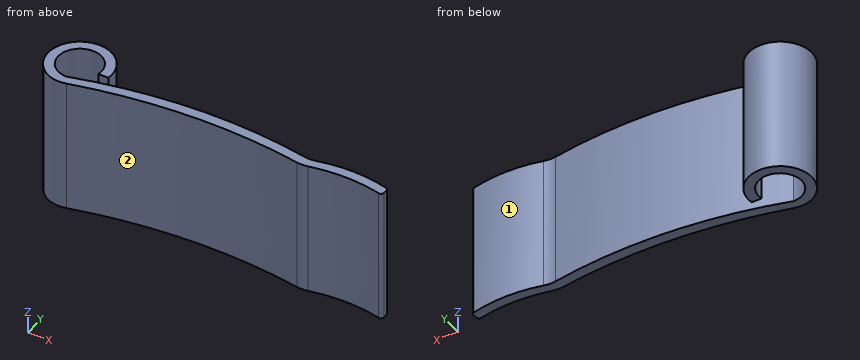
from build123d import *

# Parameters (mm, degrees)
BOSS_EXTRUDE1_DEPTH = 11.811
FILLET1_R           = 2.54
FILLET2_R           = 2.54
FILLET3_R           = 2.54
FILLET4_R           = 0.254


with BuildPart() as part:
    # Sketch1 → Boss-Extrude1 (new body)
    with BuildSketch(Plane.XY):
        with BuildLine():
            Line((28.176033565, -1.032201382), (28.176033565, -1.921201382))
            ThreePointArc((28.176033565, -1.921201382), (24.613856271, -1.460610767), (21.051678976, -1.921201382))
            ThreePointArc((21.051678976, -1.921201382), (10.446405641, -1.176341171), (-0.061202039, -2.794))
            ThreePointArc((-0.061202039, -2.794), (-1.825200311, 2.116323585), (2.772672487, -0.349955666))
            Line((2.772672487, -0.349955666), (1.874071212, -0.34188023))
            ThreePointArc((1.874071212, -0.34188023), (-1.220193255, 1.462926321), (0, -1.905))
            ThreePointArc((0, -1.905), (10.542698007, -0.186192099), (21.191033565, -1.032201382))
            ThreePointArc((21.191033565, -1.032201382), (24.683533565, -0.542543055), (28.176033565, -1.032201382))
        make_face()
    extrude(amount=BOSS_EXTRUDE1_DEPTH)

    # Fillet1
    fillet1_edges = [part.edges().sort_by_distance(p)[0] for p in [
        (-0.061202039, -2.794, 5.9055),
    ]]
    fillet(fillet1_edges, radius=FILLET1_R)

    # Fillet2
    fillet2_edges = [part.edges().sort_by_distance(p)[0] for p in [
        (21.051678976, -1.921201382, 5.9055),
    ]]
    fillet(fillet2_edges, radius=FILLET2_R)

    # Fillet3
    fillet3_edges = [part.edges().sort_by_distance(p)[0] for p in [
        (21.191033565, -1.032201382, 5.9055),
    ]]
    fillet(fillet3_edges, radius=FILLET3_R)

    # Fillet4
    fillet4_edges = [part.edges().sort_by_distance(p)[0] for p in [
        (28.176033565, -1.032201382, 5.9055),
        (28.176033565, -1.921201382, 5.9055),
    ]]
    fillet(fillet4_edges, radius=FILLET4_R)


solid = part.part
The listing builds one solid part. Answer for the finished solid, in the listing's coordinates (mm). Face numbers are marked on the shaded views. Coordinates: 2 decimals unless noted, no trailing zeros. Order: outer loops, then holes, each group sorted by start corner. A loop starts at its lowest first (then second) coordinate and runs counter-clockwise, first axis right, second up.
Q1. A cutting plane is placed at A-A, the plane y = 0.55. Write down the section's boundary in (x, z), and give its area (3 significant figures).
Q2. Given P1, Ø5, axis at x = 7, z = 7.5, coming from the -Y side; P2, Ø2, axis at x = 15, z = 8.5, coming from the +Y side; P3, Ø1, axis at x = 20, y = 1.5, coming from the -Z side; P4, Ø6, axis at x = 2.5, z = 6, coming from the +Y side, each flat-ended and moving along its own axis, determine where each tip first touches the part or whether it passes through.
Q3. Consider line 1 (Y direction, x = 0, z = 5) (3 decimals); line 2 (X direction, y = 0, z = 8.25) (3 decimals); line 3 (Y direction, x = 12.5, z = 9.25). Determine where each line is inside the solid, lowest interval first.
Q4. A cutting plane is placed at C-C, the plane y = 2.25. Write down the section's boundary in (x, z), and give its area (3 significant figures).
Q5. A cutting plane is placed at B-B, the plane x = 22. Write down the section's boundary in (y, z), and give its area (3 significant figures).
Q6. For a pull along X with two mould halves and no side action, classify the marked faces 1 and 2 as pulls with the +X half, pulls with the -X half, needs draft (parallel to the pull), parting line crosses it, or undercut.
Answers follow:
1. outline: (-2.74, 0) - (-1.82, 0) - (-1.82, 11.81) - (-2.74, 11.81) - close; (1.82, 0) - (2.74, 0) - (2.74, 11.81) - (1.82, 11.81) - close
1. area: 21.6 mm2
2. P1: stops at y = -1.8
2. P2: stops at y = -0.18
2. P3: passes through
2. P4: stops at y = 2.79
3. line 1: y = -2.729 to -1.905, 1.905 to 2.795
3. line 2: x = -2.795 to -1.905, 1.905 to 2.795
3. line 3: y = -1.14 to -0.15
4. outline: (-1.66, 0) - (1.66, 0) - (1.66, 11.81) - (-1.66, 11.81) - close
4. area: 39.2 mm2
5. outline: (-1.71, 0) - (-0.83, 0) - (-0.83, 11.81) - (-1.71, 11.81) - close
5. area: 10.4 mm2
6. face 1: undercut
6. face 2: undercut
